from build123d import *

# Parameters (mm, degrees)
AUFSATZ_LINEAR_AUSTRAGEN1_DEPTH             = 15
AUFSATZ_LINEAR_AUSTRAGEN4_DEPTH             = 1.5
AUFSATZ_LINEAR_AUSTRAGEN4_DIRECTION_2_REACH = 78.164


with BuildPart() as part:
    # Skizze1 → Aufsatz-Linear austragen1 (new body)
    with BuildSketch(Plane.XY):
        Polygon((-74, 0), (-74, -10), (-56, -10), (-56, -5), (56, -5), (56, -10), (74, -10), (74, 0), align=None)
    extrude(amount=AUFSATZ_LINEAR_AUSTRAGEN1_DEPTH)

    # Skizze5 → Aufsatz-Linear austragen4 (add)
    with BuildSketch(Plane.XZ.offset(10)):
        Polygon((56, 0), (55, 0), (55, -1), (56, -1), (75, -1), (75, 16), (56, 16), (55, 16), (55, 15), (56, 15), (74, 15), (74, 0), align=None)
    aufsatz_linear_austragen4 = extrude(amount=AUFSATZ_LINEAR_AUSTRAGEN4_DEPTH)

    # Aufsatz-Linear austragen4 direction 2: up to this face of the body (flat: up to its plane)
    aufsatz_linear_austragen4_direction_2_end = Plane(part.part.faces().sort_by_distance((0, 0, 7.5))[0])
    # Skizze5 → Aufsatz-Linear austragen4 direction 2 (add, up to the picked face)
    with BuildSketch(Plane.XZ.offset(10), mode=Mode.PRIVATE) as aufsatz_linear_austragen4_direction_2_sk1:
        Polygon((56, 0), (55, 0), (55, -1), (56, -1), (75, -1), (75, 16), (56, 16), (55, 16), (55, 15), (56, 15), (74, 15), (74, 0), align=None)
    aufsatz_linear_austragen4_direction_2_tool1 = split(extrude(aufsatz_linear_austragen4_direction_2_sk1.sketch, amount=-AUFSATZ_LINEAR_AUSTRAGEN4_DIRECTION_2_REACH, mode=Mode.PRIVATE), bisect_by=aufsatz_linear_austragen4_direction_2_end, keep=Keep.BOTH, mode=Mode.PRIVATE)
    aufsatz_linear_austragen4_direction_2 = aufsatz_linear_austragen4_direction_2_tool1.solids().sort_by(Axis((55.5, -10, -0.262488), (0, 1, 0)))[0]
    add(aufsatz_linear_austragen4_direction_2)

    # Spiegeln1: Aufsatz-Linear austragen4, Aufsatz-Linear austragen4 direction 2 across plane
    add(aufsatz_linear_austragen4.mirror(Plane(origin=(0, 0, 0), x_dir=(0, 0, 1), z_dir=(1, 0, 0))))
    add(aufsatz_linear_austragen4_direction_2.mirror(Plane(origin=(0, 0, 0), x_dir=(0, 0, 1), z_dir=(1, 0, 0))))


solid = part.part
Verification items for the finished model (mm, model axes). A direction names the side the tool comes from. Give positions to 0.01 mm unless a question says otherwise; leave off trailing zeros. Loops run counter-clockwise (first coordinate to the right, second up) from the corner with the lowest first, then second, coordinate; pieces in that order, holes last. Notation, with made-up numbers: (38, 74) - (77, 74) arc R27 cw to (77, 110) - close; hole circle Ø10 at (69, -6.5). An arc over 180 degrees is marked (long way). Write each question's results on one line, items separated by ' | '.
1) Sectioned sample at C-C on z = 13.25. Record the boundary of the cut face in (x, y).
Solution:
outline: (-75, -11.5) - (-74, -11.5) - (-74, -10) - (-56, -10) - (-56, -5) - (56, -5) - (56, -10) - (74, -10) - (74, -11.5) - (75, -11.5) - (75, 0) - (-75, 0) - close
2) Sectioned sample at A-A on y = -7.75. Record the boundary of the cut face in (x, z), plus the area to 3 significant figures.
Solution:
outline: (-75, -1) - (-55, -1) - (-55, 0) - (-56, 0) - (-56, 15) - (-55, 15) - (-55, 16) - (-75, 16) - close; (55, -1) - (75, -1) - (75, 16) - (55, 16) - (55, 15) - (56, 15) - (56, 0) - (55, 0) - close | area: 650 mm2
3) Sectioned sample at D-D on x = -18.5. Record the boundary of the cut face in (y, z).
Solution:
outline: (-5, 0) - (0, 0) - (0, 15) - (-5, 15) - close
4) Mould release check, pull along X, two halves, no side actions. Record for faces 1 (the flat face through (75, -6, 7)), 2 (the flat face through (56, -7, 7)), 3 (the flat face through (65, -6, -1)): pulls with the +X half, pulls with the -X half, needs draft (parallel to the pull), parting line crosses it, or undercut.
Solution:
face 1: pulls with the +X half | face 2: undercut | face 3: needs draft
5) Material ranges on L1, parallel to X at y = -6.75, z = 1.5; L2, parallel to Y at x = 8, z = 1.25; L3, parallel to Z at x = -14, y = -4.75, recorded low to high. Write a range as from..to.
Solution:
L1: -75..-56, 56..75 | L2: -5..0 | L3: 0..15
6) Depth check by flat-ended pin: P1, Ø2, axis at x = -40.5, z = 3.5, coming from the +Y side; P2, Ø4, axis at x = -52, y = -7.5, coming from the +Z side; P3, Ø7.5, axis at x = -21, z = 7, coming from the -Y side; P4, Ø2.5, axis at x = -16.5, y = -3, coming from the +Z side. Enter the tip coordinate at first touch or a pass-through.
Solution:
P1: y = 0 | P2: through | P3: y = -5 | P4: z = 15
7) Tool access check on faces 4 (the flat face through (-1, -2, 0)), 5 (the flat face through (-1, -2, 15)), 6 (the flat face through (63.8, -10.4, 0)). Record the directions out of +Z, -Z, +X, -X, +Y, -Y that give a thin tool (end or side, any length) a straight path to the whole face; none if there is none.
Solution:
face 4: -Z, +Y, -Y | face 5: +Z, +Y, -Y | face 6: -Y
8) Sectioned sample at B-B on x = -62. Record the boundary of the cut face in (y, z).
Solution:
outline: (-11.5, -1) - (0, -1) - (0, 16) - (-11.5, 16) - (-11.5, 15) - (-10, 15) - (-10, 0) - (-11.5, 0) - close
